from build123d import *

# Parameters (mm, degrees)
F0_W     = 100
F0_H     = 50
F1_DEPTH = 30
F2_W     = 50
F2_H     = 50
F3_DEPTH = 50
F5_DEPTH = 50
F7_DEPTH = 30


with BuildPart() as f1:
    # F0 (on Top) → F1 (new body)
    with BuildSketch(Plane.XY):
        with Locations((50, 25)):
            Rectangle(F0_W, F0_H)
    extrude(amount=F1_DEPTH)

    # F2 (on face) → F3 (join)
    with BuildSketch(Plane.XY.offset(30)):
        with Locations((25, 25)):
            Rectangle(F2_W, F2_H)
    extrude(amount=F3_DEPTH)

    # F4 (on face) → F5 (cut, through all)
    with BuildSketch(Plane.XZ):
        Polygon((20, 80), (0, 80), (0, 60), align=None)
    extrude(amount=-F5_DEPTH, mode=Mode.SUBTRACT)

    # F6 (on face) → F7 (cut, through all)
    with BuildSketch(Plane(origin=(0, 0, 0), x_dir=(1, 0, 0), z_dir=(0, 0, -1))):
        with BuildLine():
            Line((75, -25), (67.5, -25))
            ThreePointArc((67.5, -25), (69.696699, -30.303301), (75, -32.5))
            Line((75, -32.5), (75, -25))
        make_face()
        with BuildLine():
            ThreePointArc((82.5, -25), (75, -17.5), (67.5, -25))
            Line((67.5, -25), (75, -25))
            Line((75, -25), (75, -32.5))
            ThreePointArc((75, -32.5), (80.303301, -30.303301), (82.5, -25))
        make_face()
    extrude(amount=-F7_DEPTH, mode=Mode.SUBTRACT)


solid = f1.part
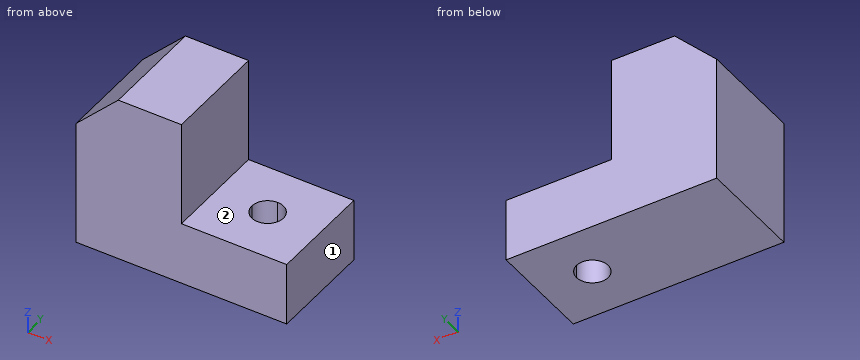
Input: part model. Units: mm. Frame: model coordinates. Face numbers are marked on the shaded views. A direction names the side the tool comes from. Coordinates: 2 decimals unless noted, no trailing zeros. Order: outer loops, then holes, each group sorted by start corner. A loop starts at its lowest first (then second) coordinate and runs counter-clockwise, first axis right, second up. Notation, with made-up numbers: M 73,32.5 L 87,32.5 A21 cw 87,65.5 Z; hole C 71,89 d5. An arc over 180 degrees is marked long. One line per question, with ' | ' between items.
Item 1: Section B-B (z = 17.5). Output: boundary loops of the cut face in (x, y), then the cut area to 3 significant figures.
Geometry results:
outline: M 0,0 L 100,0 L 100,50 L 0,50 Z; hole C 75,25 d15 | area: 4,820 mm^2
Item 2: Pin query (flat end, axial travel): pin 1 (4 mm diameter, centred on y = 39, z = 24.5, fed in from -X); pin 2 (25 mm diameter, centred on y = 30, z = 54, fed in from +X). Return the tip coordinate at first contact, or that it passes through.
Geometry results:
pin 1: stops at x = 0 | pin 2: stops at x = 50
Item 3: Reachability of the marked faces 1 and 2 from +Z, -Z, +X, -X, +Y, -Y: full face, straight path, thin tool, end or side. Return the list, or none.
Geometry results:
face 1: +Z, -Z, +X, +Y, -Y | face 2: +Z, +X, +Y, -Y
Item 4: Section D-D (x = 53). Output: boundary loops of the cut face in (y, z), then the cut area to 3 significant figures.
Geometry results:
outline: M 0,0 L 50,0 L 50,30 L 0,30 Z | area: 1,500 mm^2
Item 5: Ray query, line 1 along Z through (x, y) = (93, 31); line 2 along X through (y, z) = (11, 33); line 3 along Y through (x, z) = (74, 28). Return the intervals inside material, ascending.
Geometry results:
line 1: z = 0 to 30 | line 2: x = 0 to 50 | line 3: y = 0 to 17.57, 32.43 to 50
Item 6: Section C-C (y = 47.5). Output: boundary loops of the cut face in (x, z), then the cut area to 3 significant figures.
Geometry results:
outline: M 0,0 L 100,0 L 100,30 L 50,30 L 50,80 L 20,80 L 0,60 Z | area: 5,300 mm^2
Item 7: Section A-A (y = 20.5). Output: boundary loops of the cut face in (x, z).
Geometry results:
outline: M 0,0 L 69,0 L 69,30 L 50,30 L 50,80 L 20,80 L 0,60 Z; M 81,0 L 100,0 L 100,30 L 81,30 Z
